Design review of the part built by this model. Coordinates are the model's own, in mm. A direction names the side the tool comes from. Coordinates: 2 decimals unless noted, no trailing zeros. Loops run counter-clockwise (first coordinate to the right, second up) from the corner with the lowest first, then second, coordinate; pieces in that order, holes last. Notation, with made-up numbers: (-3, 87) -> (30, 87) arc R19 ccw to (30, 123) -> close; hole circle Ø7 at (64, 14.5). An arc over 180 degrees is marked (long way). One line per item, written item: value. Start each with the question number.
1. Insertion check: pin 1 (1.2 mm diameter, centred on x = -21.5, y = 1.5, fed in from +Z); pin 2 (1.2 mm diameter, centred on x = 97, y = 2, fed in from -Z); pin 3 (1 mm diameter, centred on y = 2.5, z = -97.5, fed in from +X). Each pin has a flat end and moves straight along its axis. Give the tip position at first contact, or say it passes through.
2. For probe 1 along X at (y, z) = (3.05, -19); probe 2 along X at (y, z) = (1, -115); probe 3 along Z at (x, y) = (49, 0.45), list the stretches that pass through material, from the lowest coordinate up.
3. Add section C-C on z = -115. Write out the cut boundary in (x, y), plus the area to 3 significant figures.
4. Draft analysis for pull direction Z (two halves, no side actions). For faces 4 (the flat face through (55, 2, 0)), 5 (the flat face through (-98, 2, -60)), 6 (the flat face through (96.094, 2, -17)), state which applies: pulls with the +Z half, pulls with the -Z half, needs draft (parallel to the pull), parting line crosses it, or undercut.
5. Add section B-B on z = -19. Write out the cut boundary in (x, y).
6. Add section D-D on y = 1.95. Give the number of separate pieces and of enclosed holes in the cut face, plus the area to 3 significant figures.
7. Machinability: for faces 1 (the flat face through (1, 2, -14)), 2 (the flat face through (-80, 2, -4)), 3 (the flat face through (98, 2, -30)), which of the approach directions +Z, -Z, +X, -X, +Y, -Y give a long, thin tool a straight path to every point of the face, cutting with its end or side? Answer none if there is none.
8. Add section A-A on x = -47.5. Write out the cut boundary in (y, z).
```python
from build123d import *

# Parameters (mm, degrees)
RESSALTO_EXTRUS_O1_DEPTH = 4
ESBO_O2_W                = 35
ESBO_O2_H                = 4
ESBO_O2_W_2              = 3.874378487
ESBO_O2_H_2              = 26.000016438
CORTE_EXTRUS_O1_DEPTH    = 5
CORTE_EXTRUS_O5_REACH    = 6
ESBO_O6_W                = 32.376232368
ESBO_O6_H                = 43.313616366
ESBO_O3_W                = 192.251243026
ESBO_O3_H                = 15
CORTE_EXTRUS_O3_DEPTH    = 5
FURO_COM_FOLGA_DE_M41_D  = 4.5
ESBO_O5_R                = 2.25
CORTE_EXTRUS_O4_DEPTH    = 5


with BuildPart() as part:
    # Esboço1 → Ressalto-extrusão1 (new body)
    with BuildSketch(Plane(origin=(0, 0, 0), x_dir=(1, 0, 0), z_dir=(0, 1, 0))):
        Polygon((-100.157081707, 150), (-100.000054794, 0), (100.000054794, 0), (99.843027881, 150), align=None)
    extrude(amount=RESSALTO_EXTRUS_O1_DEPTH)

    # Esboço2 → Corte-extrusão1 (cut, through all)
    with BuildSketch(Plane(origin=(0, 4, 0), x_dir=(1, 0, 0), z_dir=(0, 1, 0))):
        Polygon((-100.125676325, 120), (-96.157081707, 120), (-96.157081707, 150), (-100.157081707, 150), align=None)
        Polygon((-100.062865577, 60.000016438), (-96.157081707, 60.000016438), (-96.157081707, 90), (-100.094270942, 90), align=None)
        Polygon((-100.004242179, 4), (-96.157081707, 4), (-96.157081707, 30.000016438), (-100.031460194, 30.000016438), align=None)
        Polygon((-100.000054794, 0), (-65.031460194, 0), (-65.031460194, 4), (-96.157081707, 4), (-100.004242179, 4), align=None)
        with Locations((-27.531460194, 2)):
            Rectangle(ESBO_O2_W, ESBO_O2_H)
        with Locations((27.468539806, 2)):
            Rectangle(ESBO_O2_W, ESBO_O2_H)
        Polygon((64.968539806, 4), (64.968539806, 0), (99.968539806, 0), (99.968539806, 4), (96.094161319, 4), align=None)
        with Locations((98.031350563, 17.000008219)):
            Rectangle(ESBO_O2_W_2, ESBO_O2_H_2)
        Polygon((96.094161319, 60.000016438), (99.937244012, 60.000016438), (99.905838646, 90), (96.094161319, 90), align=None)
        Polygon((99.843027881, 150), (96.094161319, 150), (96.094161319, 120), (99.874433264, 120), align=None)
    extrude(amount=-CORTE_EXTRUS_O1_DEPTH, mode=Mode.SUBTRACT)

    # Esboço6 → Corte-extrusão5 (cut, up to next)
    with BuildSketch(Plane(origin=(0, 4, 0), x_dir=(1, 0, 0), z_dir=(0, 1, 0)), mode=Mode.PRIVATE) as corte_extrus_o5_sk1:
        with Locations((112.282277503, 8.343208255)):
            Rectangle(ESBO_O6_W, ESBO_O6_H)
    corte_extrus_o5_tool1 = extrude(corte_extrus_o5_sk1.sketch, amount=-CORTE_EXTRUS_O5_REACH, mode=Mode.PRIVATE) & part.part
    add(corte_extrus_o5_tool1.solids().sort_by_distance((112.282278, 4, -8.343208))[0], mode=Mode.SUBTRACT)

    # Esboço3 → Corte-extrusão3 (cut, through all)
    with BuildSketch(Plane(origin=(0, 4, 0), x_dir=(1, 0, 0), z_dir=(0, 1, 0))):
        with Locations((-0.031460194, 142.5)):
            Rectangle(ESBO_O3_W, ESBO_O3_H)
    extrude(amount=-CORTE_EXTRUS_O3_DEPTH, mode=Mode.SUBTRACT)

    # Furo com folga de M41 (through all)
    with Locations(Plane(origin=(-81.157081707, 4, -19), x_dir=(0, 0, 1), z_dir=(0, 1, 0))):
        with Locations((0, 0), (-96, 0), (-96, 162.251243026), (0, 162.251243026)):
            Hole(FURO_COM_FOLGA_DE_M41_D / 2)

    # Esboço5 → Corte-extrusão4 (cut, through all)
    with BuildSketch(Plane(origin=(0, 4, 0), x_dir=(1, 0, 0), z_dir=(0, 1, 0))):
        with Locations((-81.157081707, 19)):
            Circle(ESBO_O5_R)
        with BuildLine():
            Line((-55, 24), (55, 24))
            ThreePointArc((55, 24), (60, 19), (55, 14))
            Line((55, 14), (-55, 14))
            ThreePointArc((-55, 14), (-60, 19), (-55, 24))
        make_face()
    extrude(amount=-CORTE_EXTRUS_O4_DEPTH, mode=Mode.SUBTRACT)


solid = part.part
```
Worked answers:
1. pin 1: stops at z = -4
1. pin 2: stops at z = -120
1. pin 3: stops at x = 99.9
2. probe 1: x = -96.16 to -83.41, -78.91 to -60, 60 to 78.84, 83.34 to 96.09
2. probe 2: x = -100.12 to -83.41, -78.91 to 78.84, 83.34 to 99.88
2. probe 3: z = -135 to -24, -14 to 0
3. outline: (-100.12, 0) -> (-83.41, 0) -> (-83.41, 4) -> (-100.12, 4) -> close; (-78.91, 0) -> (78.84, 0) -> (78.84, 4) -> (-78.91, 4) -> close; (83.34, 0) -> (99.88, 0) -> (99.88, 4) -> (83.34, 4) -> close
3. area: 764 mm²
4. face 4: pulls with the +Z half
4. face 5: undercut
4. face 6: needs draft
5. outline: (-96.16, 0) -> (-83.41, 0) -> (-83.41, 4) -> (-96.16, 4) -> close; (-78.91, 0) -> (-60, 0) -> (-60, 4) -> (-78.91, 4) -> close; (60, 0) -> (78.84, 0) -> (78.84, 4) -> (60, 4) -> close; (83.34, 0) -> (96.09, 0) -> (96.09, 4) -> (83.34, 4) -> close
6. separate pieces: 1
6. enclosed holes: 5
6. area: 24,600 mm²
7. face 1: +Y, -Y
7. face 2: +Z, -X, +Y, -Y
7. face 3: +Z, +X, +Y, -Y
8. outline: (0, -135) -> (4, -135) -> (4, -24) -> (0, -24) -> close; (0, -14) -> (4, -14) -> (4, 0) -> (0, 0) -> close
